Part model, mm, in its own coordinate system. Round coordinates to 2 decimals unless told otherwise and drop trailing zeros. Loops run counter-clockwise (first coordinate to the right, second up) from the corner with the lowest first, then second, coordinate; pieces in that order, holes last. Notation, with made-up numbers: M -35.75,69 L -11.75,69 A20 cw -11.75,98 Z; hole C 23,-29 d8. An arc over 180 degrees is marked long. Put each result on its own line as item: value. Start each with the question number.
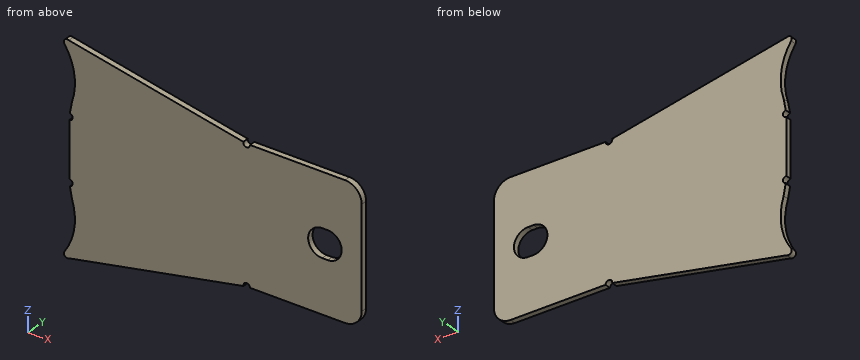
```python
from build123d import *

# Parameters (mm, degrees)
F1_DEPTH = 2.286


# Not quite as in the source:
# - ends of sketch curves that miss each other by under 0.0002 mm in the source are joined


with BuildPart() as f1:
    # F0 (on Front) → F1 (new body)
    with BuildSketch(Plane.XZ):
        with BuildLine():
            ThreePointArc((-20.1784623574, -17.2534296725), (-19.281646508, -27.4231568168), (-23.0260908036, -36.9208810585))
            ThreePointArc((-23.0260908036, -36.9208810585), (-22.9304929279, -38.4914502694), (-21.3807341969, -38.7636168977))
            Line((-21.3807341969, -38.7636168977), (44.86735167, -25.6466681175))
            ThreePointArc((44.86735167, -25.6466681175), (45.9892411408, -24.1360607291), (47.3831666, -25.4))
            Line((47.3831666, -25.4), (76.8344666, -5.3213))
            Line((76.8344666, -5.3213), (74.7770666, -5.3213))
            ThreePointArc((74.7770666, -5.3213), (69.4557666, 0), (74.7770666, 5.3213))
            Line((74.7770666, 5.3213), (76.8344666, 5.3213))
            Line((76.8344666, 5.3213), (47.3831666, 25.4))
            ThreePointArc((47.3831666, 25.4), (45.9892409445, 24.1360607483), (44.8673517466, 25.6466685044))
            Line((44.8673517466, 25.6466685044), (-21.38072359, 38.7636365822))
            ThreePointArc((-21.38072359, 38.7636365822), (-22.9304889155, 38.4914801631), (-23.026090887, 36.9209064006))
            ThreePointArc((-23.026090887, 36.9209064006), (-19.281646508, 27.4231822168), (-20.1784623574, 17.2534550725))
            Line((-20.1784623574, 17.2534550725), (-20.9658562769, 12.9963192698))
            ThreePointArc((-20.9658562769, 12.9963192698), (-19.9321396678, 11.6315268838), (-21.1968334, 10.4775))
            Line((-21.1968334, 10.4775), (-21.1968334, -10.4775))
            ThreePointArc((-21.1968334, -10.4775), (-19.9321397156, -11.6315263621), (-20.9658552466, -12.9963190792))
            Line((-20.9658552466, -12.9963190792), (-20.1784623574, -17.2534296725))
        make_face()
        with BuildLine():
            Line((76.8344666, -5.3213), (47.3831666, -25.4))
            Line((47.3831666, -25.4), (83.4257666, -25.4))
            ThreePointArc((83.4257666, -25.4), (87.9158946605, -23.5401280605), (89.7757666, -19.05))
            Line((89.7757666, -19.05), (89.7757666, 19.05))
            ThreePointArc((89.7757666, 19.05), (87.9158946605, 23.5401280605), (83.4257666, 25.4))
            Line((83.4257666, 25.4), (47.3831666, 25.4))
            Line((47.3831666, 25.4), (76.8344666, 5.3213))
            ThreePointArc((76.8344666, 5.3213), (82.1557666, 0), (76.8344666, -5.3213))
        make_face()
    extrude(amount=F1_DEPTH)


solid = f1.part
```
1. Cut at C-C, the plane x = 43.5. Give the cut face in (y, z), and give its area (3 significant figures).
2. Drop flat-ended pins along their axis: pin 1 (1 mm diameter, centred on x = 41, y = -1.5, fed in from +Z); pin 2 (1 mm diameter, centred on y = -1, z = 17, fed in from -X); pin 3 (1.5 mm diameter, centred on x = 53.5, z = -28, fed in from -Y); pin 4 (1.1 mm diameter, centred on y = -0.5, z = 3, fed in from -X). Give the stop position or say it passes through.
3. Wall check: L1, parallel to Z at x = 76, y = -0.45; L2, parallel to Z at x = 68.5, y = -1.35; L3, parallel to X at y = -0.15, z = 6. Give the ranges that are in metal, low to high.
4. Cut at A-A, the plane z = 0. Give the cut face in (x, y).
5. Cut at D-D, the plane x = -6.5. Give the cut face in (y, z), and give its area (3 significant figures).
Results list:
1. outline: M -2.29,-25.92 L 0,-25.92 L 0,25.92 L -2.29,25.92 Z
1. area: 118 mm^2
2. pin 1: stops at z = 26.51
2. pin 2: stops at x = -20.32
2. pin 3: passes through
2. pin 4: stops at x = -21.2
3. L1: z = -25.4 to -5.32, 5.32 to 25.4
3. L2: z = -25.4 to 25.4
3. L3: x = -21.2 to 89.78
4. outline: M -21.2,-2.29 L 69.46,-2.29 L 69.46,0 L -21.2,0 Z; M 82.16,-2.29 L 89.78,-2.29 L 89.78,0 L 82.16,0 Z
5. outline: M -2.29,-35.82 L 0,-35.82 L 0,35.82 L -2.29,35.82 Z
5. area: 164 mm^2
